The model under review builds one solid part; all positions refer to its coordinate system, in mm. A direction names the side the tool comes from. Coordinates: 2 decimals unless noted, no trailing zeros. Order: outer loops, then holes, each group sorted by start corner. A loop starts at its lowest first (then second) coordinate and runs counter-clockwise, first axis right, second up. Notation, with made-up numbers: (66.5, 30.5) -> (99.5, 30.5) arc R14 cw to (99.5, 45.5) -> close; hole circle Ø10 at (79, -36.5). An arc over 180 degrees is marked (long way). Answer as CSV lines item,"result". Start each with the question number.
from build123d import *

# Parameters (mm, degrees)
SKETCH_1_W                       = 230
SKETCH_1_H                       = 20
SM_BASE_FLANGE_1_DEPTH           = 1.5
SM_EDGE_FLANGE_1_STRIP_W         = 7.4732
SM_EDGE_FLANGE_1_STRIP_H         = 1.5
SM_EDGE_FLANGE_1_STRIP_CUT_DEPTH = 20
SM_EDGE_FLANGE_1_DEPTH           = 20
SM_EDGE_FLANGE_2_STRIP_W         = 7.4732
SM_EDGE_FLANGE_2_STRIP_H         = 1.5
SM_EDGE_FLANGE_2_STRIP_CUT_DEPTH = 20
SM_EDGE_FLANGE_2_DEPTH           = 20


# Sheet-metal steps are written as plain solids
with BuildPart() as part:
    # Sketch 1 → Базовая кромка1 (new body)
    with BuildSketch(Plane(origin=(0, 0, 0), x_dir=(1, 0, 0), z_dir=(0, 1, 0))):
        with Locations((115, 10)):
            Rectangle(SKETCH_1_W, SKETCH_1_H)
    extrude(amount=-SM_BASE_FLANGE_1_DEPTH)

    # Ребро-кромка1 strip (across the edge) → Ребро-кромка1 strip cut (cut)
    with BuildSketch(Plane.XY.offset(-20)):
        with Locations((-1.5, -0.75)):
            Rectangle(SM_EDGE_FLANGE_1_STRIP_W, SM_EDGE_FLANGE_1_STRIP_H)
    extrude(amount=SM_EDGE_FLANGE_1_STRIP_CUT_DEPTH, mode=Mode.SUBTRACT)

    # Ребро-кромка1 section (across the edge) → Ребро-кромка1 (add)
    with BuildSketch(Plane.XY.offset(-20)):
        with BuildLine():
            Line((0, 0.7366), (0, 33.5))
            Line((0, 33.5), (1.5, 33.5))
            Line((1.5, 33.5), (1.5, 0.7366))
            ThreePointArc((1.5, 0.7366), (1.715745145, 0.215745145), (2.2366, 0))
            Line((2.2366, 0), (2.2366, -1.5))
            ThreePointArc((2.2366, -1.5), (0.655084973, -0.844915027), (0, 0.7366))
        make_face()
    extrude(amount=SM_EDGE_FLANGE_1_DEPTH)

    # Ребро-кромка2 strip (across the edge) → Ребро-кромка2 strip cut (cut)
    with BuildSketch(Plane(origin=(230, 0, 0), x_dir=(-1, 0, 0), z_dir=(0, 0, -1))):
        with Locations((-1.5, -0.75)):
            Rectangle(SM_EDGE_FLANGE_2_STRIP_W, SM_EDGE_FLANGE_2_STRIP_H)
    extrude(amount=SM_EDGE_FLANGE_2_STRIP_CUT_DEPTH, mode=Mode.SUBTRACT)

    # Ребро-кромка2 section (across the edge) → Ребро-кромка2 (add)
    with BuildSketch(Plane(origin=(230, 0, 0), x_dir=(-1, 0, 0), z_dir=(0, 0, -1))):
        with BuildLine():
            Line((0, 0.7366), (0, 33.5))
            Line((0, 33.5), (1.5, 33.5))
            Line((1.5, 33.5), (1.5, 0.7366))
            ThreePointArc((1.5, 0.7366), (1.715745145, 0.215745145), (2.2366, 0))
            Line((2.2366, 0), (2.2366, -1.5))
            ThreePointArc((2.2366, -1.5), (0.655084973, -0.844915027), (0, 0.7366))
        make_face()
    extrude(amount=SM_EDGE_FLANGE_2_DEPTH)


solid = part.part
1) Consider section C-C (x = 205.5). Give the boundary of the cut face in (y, z).
2) Tool access review of faces 1 (the face through (230, 17, -10)), 2 (the face through (228.5, 17, -10)): name each direction out of +Z, -Z, +X, -X, +Y, -Y from which nothing blocks a thin tool from reaching the whole face with its end or side.
3) Consider section A-A (y = 24). Give the boundary of the cut face in (x, z), plus the area to 3 significant figures.
4) Insertion check: pin 1 Ø10 at (x, z) = (153, -14) entering from +Y; pin 2 Ø4 at (y, z) = (19, -2.5) entering from -X; pin 3 Ø4 at (x, y) = (95.5, 3.5) entering from +Z (3 decimals). Each pin has a flat end and moves straight along its axis. Give the tip position at first contact, or say it passes through.
5) Wall thickness on L1, parallel to X at y = 29.5, z = -5.5; L2, parallel to Y at x = 14.5, z = -14.75: over which ranges is each line inside the solid? List them lowest first. Write a range as [from, to].
6) Consider section B-B (z = -6.5). Give the boundary of the cut face in (x, y), plus the area to 3 significant figures.
Result:
1,outline,"(-1.5, -20) -> (0, -20) -> (0, 0) -> (-1.5, 0) -> close"
2,face 1,"+Z, -Z, +X, +Y, -Y"
2,face 2,"+Z, -Z, +Y"
3,outline,"(0, -20) -> (1.5, -20) -> (1.5, 0) -> (0, 0) -> close; (228.5, -20) -> (230, -20) -> (230, 0) -> (228.5, 0) -> close"
3,area,"60.0 mm2"
4,pin 1,"y = 0"
4,pin 2,"x = 0"
4,pin 3,"through"
5,L1,"[0, 1.5], [228.5, 230]"
5,L2,"[-1.5, 0]"
6,outline,"(0, 0.74) arc R2.24 ccw to (2.24, -1.5) -> (227.76, -1.5) arc R2.24 ccw to (230, 0.74) -> (230, 33.5) -> (228.5, 33.5) -> (228.5, 0.74) arc R0.74 cw to (227.76, 0) -> (2.24, 0) arc R0.74 cw to (1.5, 0.74) -> (1.5, 33.5) -> (0, 33.5) -> close"
6,area,"444 mm2"
